Autodesk Inventor part; units mm, degrees
ref_plane "YZ Plane" through (0, 0, 0) normal (1, 0, 0) x (0, 1, 0)
ref_plane "XZ Plane" through (0, 0, 0) normal (0, 1, 0) x (-1, 0, 0)
ref_plane "XY Plane" through (0, 0, 0) normal (0, 0, 1) x (1, 0, 0)
sketch "Sketch1" plane through (889, 0, -4876.8) normal (0, 1, 0) x (-1, 0, 0)
  line L0 (1778, 0) -> (1778, 9753.6)
  line L1 (1778, 0) -> (1701.8, 0)
  line L2 (1701.8, 0) -> (1701.8, 76.2)
  line L3 (1701.8, 76.2) -> (1778, 76.2)
  line L4 (1778, 76.2) -> (1778, 0)
  line L5 (889, 0) -> (889, 9753.6) construction
  line L6 (0, 9753.6) -> (1778, 9753.6)
  point P0 (0, 0)
  dimension "d0" = 76.2
  dimension "d1" = 76.2
extrude "Extrusion1" add sketch "Sketch1" along normal blind 1117.6
sketch "Sketch2" plane through (-812.8, 0, -4876.8) normal (0, 0, -1) x (-1, 0, 0)
  line L0 (19.05, 95.25) -> (57.15, 95.25)
  line L1 (57.15, 95.25) -> (57.15, 57.15)
  line L2 (57.15, 57.15) -> (19.05, 57.15)
  line L3 (19.05, 57.15) -> (19.05, 95.25)
  line L4 (19.05, 95.25) -> (57.15, 57.15) construction
  line L5 (57.15, 95.25) -> (19.05, 57.15) construction
  line L6 (19.05, 996.95) -> (57.15, 996.95)
  line L7 (57.15, 996.95) -> (57.15, 958.85)
  line L8 (57.15, 958.85) -> (19.05, 958.85)
  line L9 (19.05, 958.85) -> (19.05, 996.95)
  line L10 (19.05, 996.95) -> (57.15, 958.85) construction
  line L11 (57.15, 996.95) -> (19.05, 958.85) construction
  line L12 (76.2, 55.9997) -> (76.2, 1188.6397)
  line L13 (76.2, 0) -> (76.2, 1117.6)
  line L14 (0, 0) -> (76.2, 0)
  point P0 (-812.8, 0)
  point P1 (64.1185, -20.2003)
  point P2 (38.1, 76.2)
  point P3 (38.1, 977.9)
  dimension "d5" = 38.1
  dimension "d6" = 38.1
  dimension "d7" = 38.1
  dimension "d9" = 863.6
  dimension "d10" = 38.1
  dimension "d11" = 38.1
  dimension "d12" = 38.1
  dimension "d13" = 76.2
extrude "Extrusion2" add sketch "Sketch2" along normal blind 1981.2
sketch "Sketch3" plane through (-831.85, 95.25, -4876.8) normal (0, 1, 0) x (1, 0, 0)
  line L0 (-19.05, 7.9484) -> (-19.05, 1981.2) construction
  line L1 (345.7063, 1981.2) -> (-383.8063, 1981.2)
  line L2 (-12.7, 152.4) -> (-25.4, 152.4)
  line L3 (-25.4, 152.4) -> (-25.4, 165.1)
  line L4 (-25.4, 165.1) -> (-12.7, 165.1)
  line L5 (-12.7, 165.1) -> (-12.7, 152.4)
  line L6 (-12.7, 152.4) -> (-25.4, 165.1) construction
  line L7 (-25.4, 152.4) -> (-12.7, 165.1) construction
  line L8 (-25.4, 317.5) -> (-25.4, 330.2)
  line L9 (-25.4, 330.2) -> (-12.7, 330.2)
  line L10 (-12.7, 330.2) -> (-12.7, 317.5)
  line L11 (-12.7, 317.5) -> (-25.4, 317.5)
  line L12 (-25.4, 482.6) -> (-25.4, 495.3)
  line L13 (-25.4, 495.3) -> (-12.7, 495.3)
  line L14 (-12.7, 495.3) -> (-12.7, 482.6)
  line L15 (-12.7, 482.6) -> (-25.4, 482.6)
  line L16 (-25.4, 647.7) -> (-25.4, 660.4)
  line L17 (-25.4, 660.4) -> (-12.7, 660.4)
  line L18 (-12.7, 660.4) -> (-12.7, 647.7)
  line L19 (-12.7, 647.7) -> (-25.4, 647.7)
  line L20 (-25.4, 812.8) -> (-25.4, 825.5)
  line L21 (-25.4, 825.5) -> (-12.7, 825.5)
  line L22 (-12.7, 825.5) -> (-12.7, 812.8)
  line L23 (-12.7, 812.8) -> (-25.4, 812.8)
  line L24 (-25.4, 977.9) -> (-25.4, 990.6)
  line L25 (-25.4, 990.6) -> (-12.7, 990.6)
  line L26 (-12.7, 990.6) -> (-12.7, 977.9)
  line L27 (-12.7, 977.9) -> (-25.4, 977.9)
  line L28 (-25.4, 1143) -> (-25.4, 1155.7)
  line L29 (-25.4, 1155.7) -> (-12.7, 1155.7)
  line L30 (-12.7, 1155.7) -> (-12.7, 1143)
  line L31 (-12.7, 1143) -> (-25.4, 1143)
  line L32 (-25.4, 1308.1) -> (-25.4, 1320.8)
  line L33 (-25.4, 1320.8) -> (-12.7, 1320.8)
  line L34 (-12.7, 1320.8) -> (-12.7, 1308.1)
  line L35 (-12.7, 1308.1) -> (-25.4, 1308.1)
  line L36 (-25.4, 1473.2) -> (-25.4, 1485.9)
  line L37 (-25.4, 1485.9) -> (-12.7, 1485.9)
  line L38 (-12.7, 1485.9) -> (-12.7, 1473.2)
  line L39 (-12.7, 1473.2) -> (-25.4, 1473.2)
  line L40 (-25.4, 1638.3) -> (-25.4, 1651)
  line L41 (-25.4, 1651) -> (-12.7, 1651)
  line L42 (-12.7, 1651) -> (-12.7, 1638.3)
  line L43 (-12.7, 1638.3) -> (-25.4, 1638.3)
  line L44 (-25.4, 1803.4) -> (-25.4, 1816.1)
  line L45 (-25.4, 1816.1) -> (-12.7, 1816.1)
  line L46 (-12.7, 1816.1) -> (-12.7, 1803.4)
  line L47 (-12.7, 1803.4) -> (-25.4, 1803.4)
  line L48 (19.05, 0) -> (-57.15, 0)
  line L49 (-38.1, 0) -> (-38.1, 1981.2)
  line L50 (-38.1, 1981.2) -> (0, 1981.2)
  point P0 (831.85, -4876.8)
  point P1 (-524.2437, -132.1024)
  point P2 (-19.05, 158.75)
  dimension "d20" = 12.7
  dimension "d21" = 12.7
  dimension "d23" = 165.1
  dimension "d25" = 152.4
  dimension "d27" = 19.05
  dimension "d28" = 0
extrude "Extrusion3" add sketch "Sketch3" along normal up to surface (863.6 mm away)
properties part number "Railing" material "Iron, Wrought"
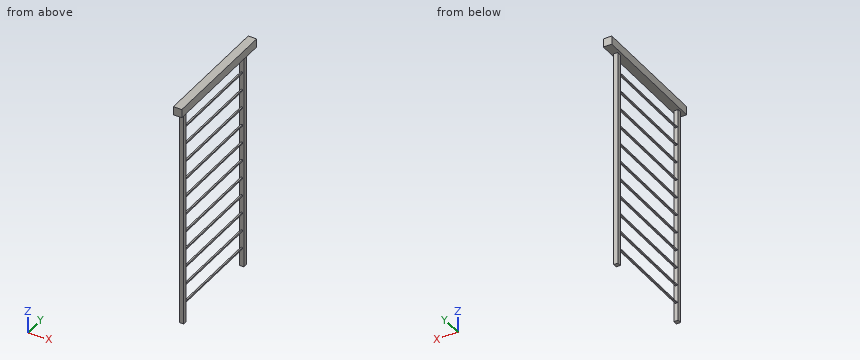
CAD build for the part. Positions are in the model's coordinates, mm. Give positions to 0.01 mm unless a question says otherwise; leave off trailing zeros. Loops run counter-clockwise (first coordinate to the right, second up) from the corner with the lowest first, then second, coordinate; pieces in that order, holes last. Notation, with made-up numbers: M 37.25,12 L 72.25,12 A16 ccw 72.25,32 Z; hole C 58,-6 d11. An arc over 180 degrees is marked long. Answer in a Markdown table with one row per item. Add a question column.
Item 1: Drop flat-ended pins along their axis: P1, Ø10, axis at y = 614.5, z = -6519, coming from the -X side; P2, Ø4, axis at x = -850, z = -5548.5, coming from the +Y side; P3, Ø4, axis at y = 736, z = -6689, coming from the +X side. Give the stop position or say it passes through.
Item 2: Band-saw the part on A-A on z = -5459.5. Give the cut face in (x, y), then the cut area to 3 significant figures.
Item 3: Band-saw the part on B-B on y = 778. Give the number of separate pieces and of enclosed holes in the cut face, then the cut area to 3 significant figures.
Item 4: Probe probe 1 along Y at (x, z) = (-869.5, -6215.5); probe 2 along Z at (x, y) = (-844, 354.5); probe 3 along X at (y, z) = (94, -5420). List the from-to ranges inside material, lowest first.
Reply:
| question | item | result |
|---|---|---|
| 1 | P1 | stops at x = -857.25 |
| 1 | P2 | stops at y = 996.95 |
| 1 | P3 | stops at x = -844.55 |
| 2 | outline | M -869.95,57.15 L -831.85,57.15 L -831.85,95.25 L -869.95,95.25 Z; M -869.95,958.85 L -831.85,958.85 L -831.85,996.95 L -869.95,996.95 Z |
| 2 | area | 2,900 mm^2 |
| 3 | separate pieces | 12 |
| 3 | enclosed holes | 0 |
| 3 | area | 7,580 mm^2 |
| 4 | probe 1 | y = 57.15 to 95.25, 958.85 to 996.95 |
| 4 | probe 2 | z = -4876.8 to -4800.6 |
| 4 | probe 3 | x = -869.95 to -831.85 |
